Input: part model. Units: mm. Frame: model coordinates. Face numbers are marked on the shaded views. A direction names the side the tool comes from. Coordinates: 2 decimals unless noted, no trailing zeros. Loops run counter-clockwise (first coordinate to the right, second up) from the corner with the lowest first, then second, coordinate; pieces in that order, holes last.
Item 1: Ray query, line 1 along Z through (x, y) = (19, 4.5) (3 decimals); line 2 along Z through (x, y) = (74, 1); line 3 along X through (y, z) = (5.25, 18.5). Return the intervals inside material, ascending.
Item 2: Section D-D on y = 2.75. Give the number of separate pieces and of enclosed holes in the cut face, and give its area (3 significant figures).
Item 3: Pull-direction query (Z, two-part tool) for the marked faces 4, 5, 6 and 7; classes: released by +Z, released by -Z, zero draft, split by the parting line, or undercut.
Item 4: Contact query for flat-ended pins moving along their axis: P1, Ø1, axis at x = 1, y = 4.5, coming from the +Z side; P2, Ø3, axis at y = 3, z = 21.5, coming from the -X side; P3, Ø4, axis at x = 96.5, z = -4.5, coming from the +Y side. Output: stop coordinate, or through.
Item 5: Reachability of the marked faces 1, 2 and 3 from +Z, -Z, +X, -X, +Y, -Y: full face, straight path, thin tool, end or side. Return the list, or none.
Item 6: Section C-C on x = 70. Return loops of the section in (y, z) (3 decimals), and give its area (3 significant figures).
Item 7: Section B-B on y = 7.5. Return loops of the section in (x, z) (3 decimals), and give its area (3 significant figures).
Item 8: Section A-A on z = 30. Return loops of the section in (x, y) (3 decimals).
```python
from build123d import *

# Parameters (mm, degrees)
SKETCH1_R           = 4.7625
SKETCH1_R_2         = 1.5
BOSS_EXTRUDE1_DEPTH = 9.525
FILLET1_R           = 3.175
FILLET2_R           = 3.175
SKETCH3_R           = 12.7
CUT_EXTRUDE2_DEPTH  = 3.175
SKETCH4_W           = 12.7
SKETCH4_H           = 25.4
CUT_EXTRUDE3_DEPTH  = 10.525
FILLET3_R           = 3.175


with BuildPart() as part:
    # Sketch1 → Boss-Extrude1 (new body)
    with BuildSketch(Plane(origin=(0, 0, 0), x_dir=(1, 0, 0), z_dir=(0, 1, 0))):
        with BuildLine():
            Line((0, 0), (38.1, 0))
            ThreePointArc((38.1, 0), (52.620300687, 4.403064286), (63.218539249, 15.261399634))
            ThreePointArc((63.218539249, 15.261399634), (67.86863694, 19.924564568), (74.228922018, 21.631986448))
            Line((74.228922018, 21.631986448), (99.628922018, 21.631986448))
            ThreePointArc((99.628922018, 21.631986448), (110.444915242, 10.815993224), (99.628922018, 0))
            Line((99.628922018, 0), (88.9, 0))
            Line((88.9, 0), (114.3, -38.1))
            Line((114.3, -38.1), (6.35, -38.1))
            Line((6.35, -38.1), (6.35, -12.7))
            Line((6.35, -12.7), (0, -12.7))
            Line((0, -12.7), (0, 0))
        make_face()
        with Locations((99.628922018, 10.815993224)):
            Circle(SKETCH1_R, mode=Mode.SUBTRACT)
        with Locations((69.568539249, 15.261399634)):
            Circle(SKETCH1_R_2, mode=Mode.SUBTRACT)
        with Locations((82.268539249, 15.261399634)):
            Circle(SKETCH1_R_2, mode=Mode.SUBTRACT)
    extrude(amount=BOSS_EXTRUDE1_DEPTH)

    # Fillet1
    fillet1_edges = [part.edges().sort_by_distance(p)[0] for p in [
        (88.9, 4.7625, 0),
    ]]
    fillet(fillet1_edges, radius=FILLET1_R)

    # Fillet2
    fillet2_edges = [part.edges().sort_by_distance(p)[0] for p in [
        (6.35, 4.7625, 12.7),
    ]]
    fillet(fillet2_edges, radius=FILLET2_R)

    # Sketch3 → Cut-Extrude2 (cut)
    with BuildSketch(Plane(origin=(0, 9.525, 0), x_dir=(1, 0, 0), z_dir=(0, 1, 0))):
        with Locations((99.628922018, 10.815993224)):
            Circle(SKETCH3_R)
    extrude(amount=-CUT_EXTRUDE2_DEPTH, mode=Mode.SUBTRACT)

    # Sketch4 → Cut-Extrude3 (cut, through all)
    with BuildSketch(Plane(origin=(0, 9.525, 0), x_dir=(1, 0, 0), z_dir=(0, 1, 0))):
        with Locations((19.05, -22.225)):
            Rectangle(SKETCH4_W, SKETCH4_H)
    extrude(amount=-CUT_EXTRUDE3_DEPTH, mode=Mode.SUBTRACT)

    # Fillet3
    fillet3_edges = [part.edges().sort_by_distance(p)[0] for p in [
        (12.7, 4.7625, 9.525),
        (25.4, 4.7625, 9.525),
        (25.4, 4.7625, 34.925),
        (12.7, 4.7625, 34.925),
    ]]
    fillet(fillet3_edges, radius=FILLET3_R)


solid = part.part
```
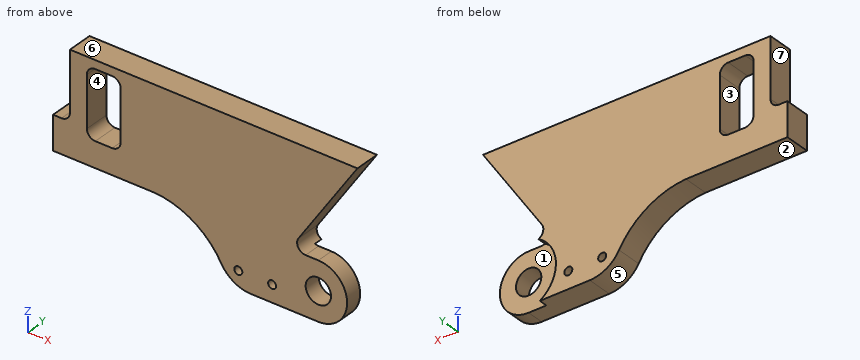
Results found:
1. line 1: z = 0 to 9.525, 34.925 to 38.1
1. line 2: z = -21.63 to 38.1
1. line 3: x = 6.35 to 12.7, 25.4 to 101.23
2. separate pieces: 1
2. enclosed holes: 4
2. area: 4,390 mm2
3. face 4: undercut
3. face 5: released by -Z
3. face 6: released by +Z
3. face 7: zero draft
4. P1: stops at z = 12.7
4. P2: stops at x = 6.35
4. P3: stops at y = 6.35
5. face 1: +X, +Y
5. face 2: -Z, -X, +Y, -Y
5. face 3: +Y, -Y
6. outline: (0, -20.907) - (9.525, -20.907) - (9.525, -16.698) - (0, -16.698) - close; (0, -13.825) - (9.525, -13.825) - (9.525, 38.1) - (0, 38.1) - close
6. area: 535 mm2
7. outline: (0, 0) - (38.1, 0) arc R30.48 cw to (63.219, -15.261) arc R12.7 ccw to (74.229, -21.632) - (92.973, -21.632) arc R12.7 cw to (93.486, 0.3) arc R3.175 cw to (92.191, 4.936) - (114.3, 38.1) - (6.35, 38.1) - (6.35, 15.875) arc R3.175 cw to (3.175, 12.7) - (0, 12.7) - close; hole (12.7, 12.7) arc R3.175 ccw to (15.875, 9.525) - (22.225, 9.525) arc R3.175 ccw to (25.4, 12.7) - (25.4, 31.75) arc R3.175 ccw to (22.225, 34.925) - (15.875, 34.925) arc R3.175 ccw to (12.7, 31.75) - close; hole circle Ø3 at (69.569, -15.261); hole circle Ø3 at (82.269, -15.261)
7. area: 4,040 mm2
8. outline: (6.35, 0) - (12.7, 0) - (12.7, 9.525) - (6.35, 9.525) - close; (25.4, 0) - (108.9, 0) - (108.9, 9.525) - (25.4, 9.525) - close
